The listing builds one solid part. Answer for the finished solid, in the listing's coordinates (mm). A direction names the side the tool comes from. Coordinates: 2 decimals unless noted, no trailing zeros. Write each loop counter-clockwise with the first axis right and the second up, starting at its lowest first coordinate (ties: lowest second). Pieces come first, ordered by that corner, then holes. Notation, with made-up numbers: M 59,60.25 L 115,60.25 A25 cw 115,88.25 Z; hole C 17.5,52.5 d11. An arc over 180 degrees is marked long. Write item = value, one per line. Start each with the question number.
```python
from build123d import *

# Parameters (mm, degrees)
SKETCH_3_W          = 126
SKETCH_3_H          = 66
SKETCH_3_W_2        = 120
SKETCH_3_H_2        = 60
EXTRUDE_2_DEPTH     = 35
SKETCH_4_W          = 6
SKETCH_4_H          = 3
SKETCH_4_W_2        = 5
SKETCH_4_W_3        = 3
SKETCH_4_H_2        = 5
EXTRUDE_3_DEPTH     = 35
SKETCH_5_W          = 120
SKETCH_5_H          = 60
CUT_EXTRUDE_1_DEPTH = 3
EXTRUDE_4_DEPTH     = 32
SKETCH_7_W          = 126
SKETCH_7_H          = 66
EXTRUDE_5_DEPTH     = 3
SKETCH_8_W          = 3
SKETCH_8_H          = 2
EXTRUDE_6_DEPTH     = 114
SKETCH_10_R         = 2.25
CUT_EXTRUDE_2_DEPTH = 3


with BuildPart() as part:
    # Эскиз3 → Бобышка-Вытянуть2 (new body)
    with BuildSketch(Plane(origin=(0, 0, 0), x_dir=(1, 0, 0), z_dir=(0, 1, 0))):
        with Locations((63, 33)):
            Rectangle(SKETCH_3_W, SKETCH_3_H)
        with Locations((63, 33)):
            Rectangle(SKETCH_3_W_2, SKETCH_3_H_2, mode=Mode.SUBTRACT)
    extrude(amount=EXTRUDE_2_DEPTH)

    # Эскиз4 → Бобышка-Вытянуть3 (add)
    with BuildSketch(Plane(origin=(0, 35, 0), x_dir=(1, 0, 0), z_dir=(0, 1, 0))):
        with Locations((6, 19.5)):
            Rectangle(SKETCH_4_W, SKETCH_4_H)
        with Locations((6, 46.5)):
            Rectangle(SKETCH_4_W, SKETCH_4_H)
        with Locations((120.5, 33)):
            Rectangle(SKETCH_4_W_2, SKETCH_4_H)
        with Locations((24.5, 60.5)):
            Rectangle(SKETCH_4_W_3, SKETCH_4_H_2)
        with Locations((101.5, 60.5)):
            Rectangle(SKETCH_4_W_3, SKETCH_4_H_2)
        with Locations((101.5, 5.5)):
            Rectangle(SKETCH_4_W_3, SKETCH_4_H_2)
        with Locations((24.5, 5.5)):
            Rectangle(SKETCH_4_W_3, SKETCH_4_H_2)
    extrude(amount=-EXTRUDE_3_DEPTH)

    # Эскиз5 → Вырез-Вытянуть1 (cut)
    with BuildSketch(Plane(origin=(0, 35, 0), x_dir=(1, 0, 0), z_dir=(0, 1, 0))):
        with Locations((63, 33)):
            Rectangle(SKETCH_5_W, SKETCH_5_H)
    extrude(amount=-CUT_EXTRUDE_1_DEPTH, mode=Mode.SUBTRACT)

    # Эскиз6 → Бобышка-Вытянуть4 (add)
    with BuildSketch(Plane.XZ):
        with BuildLine():
            Line((3, -63), (9, -63))
            Line((9, -63), (9, -61))
            ThreePointArc((9, -61), (7.828427125, -58.171572875), (5, -57))
            Line((5, -57), (3, -57))
            Line((3, -57), (3, -63))
        make_face()
        with BuildLine():
            Line((3, -9), (5, -9))
            ThreePointArc((5, -9), (7.828427125, -7.828427125), (9, -5))
            Line((9, -5), (9, -3))
            Line((9, -3), (3, -3))
            Line((3, -3), (3, -9))
        make_face()
        with BuildLine():
            Line((123, -3), (117, -3))
            Line((117, -3), (117, -5))
            ThreePointArc((117, -5), (118.171572875, -7.828427125), (121, -9))
            Line((121, -9), (123, -9))
            Line((123, -9), (123, -3))
        make_face()
        with BuildLine():
            Line((123, -57), (121, -57))
            ThreePointArc((121, -57), (118.171572875, -58.171572875), (117, -61))
            Line((117, -61), (117, -63))
            Line((117, -63), (123, -63))
            Line((123, -63), (123, -57))
        make_face()
    extrude(amount=-EXTRUDE_4_DEPTH)

    # Эскиз7 → Бобышка-Вытянуть5 (add)
    with BuildSketch(Plane.XZ):
        with Locations((63, -33)):
            Rectangle(SKETCH_7_W, SKETCH_7_H)
    extrude(amount=EXTRUDE_5_DEPTH)

    # Эскиз8 → Бобышка-Вытянуть6 (add)
    with BuildSketch(Plane(origin=(9, 0, 0), x_dir=(0, 0, -1), z_dir=(1, 0, 0))):
        with Locations((19.5, 1)):
            Rectangle(SKETCH_8_W, SKETCH_8_H)
        with Locations((46.5, 1)):
            Rectangle(SKETCH_8_W, SKETCH_8_H)
    extrude(amount=EXTRUDE_6_DEPTH)

    # Эскиз10 → Вырез-Вытянуть2 (cut)
    with BuildSketch(Plane.ZY):
        with Locations((-53, 20)):
            Circle(SKETCH_10_R)
        with Locations((-13, 20)):
            Circle(SKETCH_10_R)
    extrude(amount=-CUT_EXTRUDE_2_DEPTH, mode=Mode.SUBTRACT)


solid = part.part
```
1. Each of these flat-tipped pins is pushed along its axis until it touches: pin 1 (4 mm diameter, centred on x = 79.5, z = -50.5, fed in from +Y); pin 2 (0.9 mm diameter, centred on x = 121, z = -33.5, fed in from +Y). Where does it stop, or does it pass through?
2. For faces 4 (the face through (1.479, 17.804, -13.488)), 5 (the face through (62, 16, 0)), 6 (the face through (118, 16, -33)), determine the directions among +Z, -Z, +X, -X, +Y, -Y from which every point of the face is accessible in a straight line to the end or side of a thin tool.
3. The part is cut by section A-A, the plane z = -53. Write down the section's boundary in (x, y).
4. The part is cut by section C-C, the plane z = -43. Write down the section's boundary in (x, y), and give its area (3 significant figures).
5. For a pull along X with two mould halves and no side action, classify faces 1 (the face through (62, 0, -10)), 2 (the face through (58, 35, -1)), 3 (the face through (126, 16, -33)) as pulls with the +X half, pulls with the -X half, needs draft (parallel to the pull), parting line crosses it, or undercut.
6. Straight lines are drawn through the part: L1, parallel to Z at x = 111, y = 0.5; L2, parallel to Y at x = 2.45, z = -13; L3, parallel to X at y = 9, z = -5.5. For each, find the intervals that lie inside material, in ascending order. Write a range as [from, to].
7. The part is cut by section B-B, the plane x = 49.5. Write down the section's boundary in (y, z), and give its area (3 significant figures).
Solution:
q1.pin_1 = 0
q1.pin_2 = 32
q2.face_4 = -X
q2.face_5 = +Z, +X, -X, +Y, -Y
q2.face_6 = +Y
q3.outline = M 0,-3 L 126,-3 L 126,35 L 123,35 L 123,0 L 3,0 L 3,17.75 L 0,17.75 Z; M 0,22.25 L 3,22.25 L 3,35 L 0,35 Z
q4.outline = M 0,-3 L 126,-3 L 126,35 L 123,35 L 123,0 L 3,0 L 3,35 L 0,35 Z
q4.area = 588 mm^2
q5.face_1 = undercut
q5.face_2 = needs draft
q5.face_3 = pulls with the +X half
q6.L1 = [-66, -63], [-48, -45], [-21, -18], [-3, 0]
q6.L2 = [-3, 17.75], [22.25, 35]
q6.L3 = [0, 8.97], [23, 26], [100, 103], [117.03, 126]
q7.outline = M -3,-66 L 35,-66 L 35,-63 L 0,-63 L 0,-48 L 2,-48 L 2,-45 L 0,-45 L 0,-21 L 2,-21 L 2,-18 L 0,-18 L 0,-3 L 35,-3 L 35,0 L -3,0 Z
q7.area = 420 mm^2
